Part model, mm, in its own coordinate system. A direction names the side the tool comes from. Give positions to 0.01 mm unless a question says otherwise; leave off trailing zeros. Order: outer loops, then holes, each group sorted by start corner. A loop starts at its lowest first (then second) coordinate and runs counter-clockwise, first axis right, second up.
1. Slice it at B-B on y = -3. List the corners of the cut face in (x, z), and give its area (3 significant figures).
2. Probe line 1 (Y direction, x = -10.5, z = 3.5); line 2 (X direction, y = 11, z = -1); line 3 (Y direction, x = -21.5, z = 26.5). List the from-to ranges inside material, lowest first.
3. Slice it at D-D on z = 31. List the corners of the cut face in (x, y), and give its area (3 significant figures).
4. Slice it at C-C on z = 20. List the corners of the cut face in (x, y), and give its area (3 significant figures).
5. Which spindle directions (+Z, -Z, +X, -X, +Y, -Y) get a long thin tool onto all of the face, cutting with end or side? Do faces 1 (the flat face through (-20, -29, 19)), 2 (the flat face through (-29, 0, 1.5)), 3 (the flat face through (25.07, -26.805, 15.767)). Say none if no direction does.
6. Slice it at A-A on x = -5. List the corners of the cut face in (y, z).
7. Mould opens along Y. For faces 4 (the flat face through (-25.07, -25.44, 30.37)), 5 (the flat face through (0, 25.5, -1)), 6 (the flat face through (-21, 0, 2)), 7 (the flat face through (-25.07, -31.063, 19.192)) say: +Y half, -Y half, draft (parallel to the pull), parting line (faces both ways), or undercut.
8. Drop flat-ended pins along their axis: pin 1 Ø2 at (y, z) = (9.5, -1) entering from -X; pin 2 Ø3 at (x, z) = (-22.5, 11.5) entering from +Y; pin 3 Ø21 at (x, y) = (-0.5, -5.5) entering from +Z; pin 4 Ø2 at (x, z) = (-2.5, -1) entering from +Y. Give the stop position or say it passes through.
from build123d import *

# Parameters (mm, degrees)
EXTRUDE_1_DEPTH      = 4.5
EXTRUDE_1_DEPTH_BACK = 2
SKETCH_1_W           = 60
SKETCH_1_H           = 70
SKETCH_1_W_2         = 41
SKETCH_1_H_2         = 51
SKETCH_2_W           = 42
SKETCH_2_H           = 52
CUT_EXTRUDE_2_DEPTH  = 47.316843588
EXTRUDE_2_DEPTH      = 10


with BuildPart() as part:
    # Эскиз1 → Бобышка-Вытянуть1 (new, two sides: drawn at the far end of the back side and taken through both)
    with BuildSketch(Plane.XY.offset(-EXTRUDE_1_DEPTH_BACK)):
        Rectangle(SKETCH_1_W, SKETCH_1_H)
        Rectangle(SKETCH_1_W_2, SKETCH_1_H_2, mode=Mode.SUBTRACT)
    extrude(amount=EXTRUDE_1_DEPTH + EXTRUDE_1_DEPTH_BACK)

    # Эскиз2 → Вырез-Вытянуть2 (cut, through all)
    with BuildSketch(Plane(origin=(0, 0, 0), x_dir=(-1, 0, 0), z_dir=(0, 0, -1))):
        Rectangle(SKETCH_2_W, SKETCH_2_H)
    extrude(amount=-CUT_EXTRUDE_2_DEPTH, mode=Mode.SUBTRACT)

    # Вырез-По траектории1: sweep along a path in Эскиз4
    with BuildLine(Plane(origin=(0, 0, -2), x_dir=(-1, 0, 0), z_dir=(0, 0, -1))) as sweep_1_path:
        Line((-30, 35), (-30, -35))
        Line((-30, -35), (30, -35))
        Line((30, -35), (30, 35))
        Line((30, 35), (-30, 35))
    # Эскиз3 → Вырез-По траектории1 (sweep, cut)
    with BuildSketch(Plane(origin=(0, -35, 0), x_dir=(-1, 0, 0), z_dir=(0, -1, 0))):
        with BuildLine():
            Line((-30, 2), (-30, -1.5))
            Line((-30, -1.5), (-28.5, -1.5))
            Line((-28.5, -1.5), (-28.5, -2.5))
            Line((-28.5, -2.5), (-27, -2.5))
            Line((-27, -2.5), (-27, -2))
            ThreePointArc((-27, -2), (-25.297684645, 0.454165972), (-22.5, 1.5))
            Line((-22.5, 1.5), (-22, 1.5))
            Line((-22, 1.5), (-22, 2))
            Line((-22, 2), (-30, 2))
        make_face()
    sweep(path=sweep_1_path.line, transition=Transition.RIGHT, mode=Mode.SUBTRACT)

    # Эскиз5 → Бобышка-Вытянуть2 (add)
    with BuildSketch(Plane(origin=(30, 0, 0), x_dir=(0, 0, -1), z_dir=(1, 0, 0))):
        Polygon((-33.477774789, -27.235428647), (-4.5, -35), (-4.5, -29.823619098), (-27.354050432, -23.699894741), align=None)
    extrude_2 = extrude(amount=-EXTRUDE_2_DEPTH)

    # Зеркальное отражение1: Бобышка-Вытянуть2 across plane
    add(extrude_2.mirror(Plane(origin=(0, 0, 0), x_dir=(0, 0, 1), z_dir=(1, 0, 0))))


solid = part.part
Data:
1. outline: (-30, 1.5) - (-28.5, 1.5) - (-28.5, 2.5) - (-27, 2.5) - (-27, 2) arc R5 ccw to (-22.5, -1.5) - (-22, -1.5) - (-22, -2) - (-20.5, -2) - (-20.5, 0) - (-21, 0) - (-21, 4.5) - (-30, 4.5) - close; (20.5, -2) - (22, -2) - (22, -1.5) - (22.5, -1.5) arc R5 ccw to (27, 2) - (27, 2.5) - (28.5, 2.5) - (28.5, 1.5) - (30, 1.5) - (30, 4.5) - (21, 4.5) - (21, 0) - (20.5, 0) - close
1. area: 81.2 mm2
2. line 1: y = -35 to -26, 26 to 35
2. line 2: x = -24.42 to -20.5, 20.5 to 24.42
2. line 3: y = -29.11 to -23.93
3. outline: (-30, -27.9) - (-20, -27.9) - (-20, -25.8) - (-30, -25.8) - close; (20, -27.9) - (30, -27.9) - (30, -25.8) - (20, -25.8) - close
3. area: 41.9 mm2
4. outline: (-30, -30.85) - (-20, -30.85) - (-20, -25.67) - (-30, -25.67) - close; (20, -30.85) - (30, -30.85) - (30, -25.67) - (20, -25.67) - close
4. area: 104 mm2
5. face 1: +Z, +Y, -Y
5. face 2: -Z
5. face 3: +X, -X, +Y
6. outline: (-35, 1.5) - (-33.5, 1.5) - (-33.5, 2.5) - (-32, 2.5) - (-32, 2) arc R5 ccw to (-27.5, -1.5) - (-27, -1.5) - (-27, -2) - (-25.5, -2) - (-25.5, 0) - (-26, 0) - (-26, 4.5) - (-35, 4.5) - close; (25.5, -2) - (27, -2) - (27, -1.5) - (27.5, -1.5) arc R5 ccw to (32, 2) - (32, 2.5) - (33.5, 2.5) - (33.5, 1.5) - (35, 1.5) - (35, 4.5) - (26, 4.5) - (26, 0) - (25.5, 0) - close
7. face 4: +Y half
7. face 5: undercut
7. face 6: undercut
7. face 7: -Y half
8. pin 1: stops at x = -25.81
8. pin 2: stops at y = -27.55
8. pin 3: passes through
8. pin 4: stops at y = 30.81
